The model under review builds one solid part; all positions refer to its coordinate system, in mm. A direction names the side the tool comes from. Give positions to 0.01 mm unless a question says otherwise; leave off trailing zeros. Loops run counter-clockwise (first coordinate to the right, second up) from the corner with the lowest first, then second, coordinate; pieces in that order, holes last. Notation, with made-up numbers: M 59.5,45.25 L 108.5,45.25 A26 ccw 108.5,65.25 Z; hole C 12,74.25 d10. An arc over 180 degrees is marked long. One line per item, written item: value. Start each with the question number.
Q1. We need section B-B on x = 0. Write out the cut boundary in (y, z), plus the area to 3 significant figures.
Q2. We need section C-C on z = -78. Write out the cut boundary in (x, y), plus the area to 3 significant figures.
Q3. For faces 1 (the face through (-41.09, -8.87, -68.35)), 2 (the face through (-61, -48, -85)), 3 (the face through (4.1, -9, 20)), 4 (the face through (0, -12, -7)), list the 3-axis set-ups (+Z, -Z, +X, -X, +Y, -Y) from which the entire face can be reached by the end or side of a thin tool; tool diameter is ignored.
Q4. To check wall thickness, follow line 1 along Y through (x, z) = (-46.5, -81); line 2 along X through (y, z) = (-4.55, 19.5); line 3 along Y through (x, z) = (0, 3.5). State the ranges of each line that lie inside material, in increasing order. Write a range as from..to.
Q5. Mouldability with a two-part tool opening along Y and no side actions: class faces 5 (the face through (0, -5, 30)), 6 (the face through (-61, -30, -85)), 7 (the face through (-7, 0, -22)), 8 (the face through (-41.09, -68.87, -68.35)) as released by +Y, released by -Y, zero draft, split by the parting line, or undercut.
Q6. We need section A-A on z = 19.5. Write out the cut boundary in (x, y).
Q7. We need section D-D on y = -9. Write out the cut boundary in (x, z).
Q8. For pin 1 (2 mm diameter, centred on x = -39.5, y = -53.5, fed in from -Z); pin 2 (17.5 mm diameter, centred on x = -4, y = -33.5, fed in from +Z); pin 3 (22 mm diameter, centred on x = -58, z = -84, fed in from +Y); pin 4 (2 mm diameter, centred on x = 0, z = 15.5, fed in from -Y), all flat-tipped, find the tip position at first contact; note any pin that passes through.
```python
from build123d import *

# Parameters (mm, degrees)
SKETCH_1_W          = 16
SKETCH_1_H          = 60
EXTRUDE_1_DEPTH     = 12
EXTRUDE_2_DEPTH     = 90
SKETCH_3_W          = 16
SKETCH_3_H          = 18
CUT_EXTRUDE_2_DEPTH = 50
CUT_EXTRUDE_START   = -6
SKETCH_2_W          = 8.2
SKETCH_2_H          = 20
SKETCH_2_R          = 1.75
CUT_EXTRUDE_3_DEPTH = 6
SKETCH_2_4_R        = 1.75
CUT_EXTRUDE_4_DEPTH = 12


with BuildPart() as part:
    # Sketch 1 → Extrude 1 (new body)
    with BuildSketch(Plane(origin=(0, 0, 0), x_dir=(1, 0, 0), z_dir=(0, 1, 0))):
        Rectangle(SKETCH_1_W, SKETCH_1_H)
    extrude(amount=-EXTRUDE_1_DEPTH)

    # Sketch 1_4 → Extrude 2 (add)
    with BuildSketch(Plane(origin=(0, 0, 0), x_dir=(1, 0, 0), z_dir=(0, 1, 0))):
        Polygon((-84.604444312, 94.278760969), (-74.319842557, 106.535472059), (2.284601755, 42.25671109), (-8, 30), align=None)
        with BuildLine():
            Line((-8, 30), (8, 30))
            ThreePointArc((8, 30), (6.500924593, 36.761892188), (2.284601755, 42.25671109))
            Line((2.284601755, 42.25671109), (-8, 30))
        make_face()
    extrude(amount=-EXTRUDE_2_DEPTH)

    # Sketch 3 → Cut-Extrude 2 (cut)
    with BuildSketch(Plane(origin=(-96.071153318, 0, -80.613269316), x_dir=(-0.64278761, 0, 0.766044443), z_dir=(-0.766044443, 0, -0.64278761))):
        with Locations((-25.839032416, -9)):
            Rectangle(SKETCH_3_W, SKETCH_3_H)
        with Locations((-25.839032416, -39)):
            Rectangle(SKETCH_3_W, SKETCH_3_H)
        with Locations((-25.839032416, -69)):
            Rectangle(SKETCH_3_W, SKETCH_3_H)
    extrude(amount=-CUT_EXTRUDE_2_DEPTH, mode=Mode.SUBTRACT)

    # Sketch 2 → Cut-Extrude 3 (cut)
    with BuildSketch(Plane(origin=(0, 0, 0), x_dir=(1, 0, 0), z_dir=(0, 1, 0)).offset(CUT_EXTRUDE_START)):
        with Locations((0, -20)):
            Rectangle(SKETCH_2_W, SKETCH_2_H)
        with Locations((0, -19.5)):
            Circle(SKETCH_2_R, mode=Mode.SUBTRACT)
        with Locations((0, -15.5)):
            Circle(SKETCH_2_R, mode=Mode.SUBTRACT)
    extrude(amount=-CUT_EXTRUDE_3_DEPTH, mode=Mode.SUBTRACT)

    # Sketch 2_4 → Cut-Extrude 4 (cut)
    with BuildSketch(Plane(origin=(0, 0, 0), x_dir=(1, 0, 0), z_dir=(0, 1, 0))):
        with Locations((0, -19.5)):
            Circle(SKETCH_2_4_R)
        with Locations((0, -15.5)):
            Circle(SKETCH_2_4_R)
    extrude(amount=-CUT_EXTRUDE_4_DEPTH, mode=Mode.SUBTRACT)


solid = part.part
```
Solved:
1. outline: M -90,-44.17 L 0,-44.17 L 0,13.75 L -6,13.75 L -6,10 L -12,10 L -12,-30 L -90,-30 Z; M -6,17.25 L 0,17.25 L 0,17.75 L -6,17.75 Z; M -6,21.25 L 0,21.25 L 0,30 L -6,30 Z
1. area: 1,830 mm2
2. outline: M -65.2,-90 L -40.31,-90 L -40.31,-78 L -65.2,-78 Z; M -65.2,-60 L -40.31,-60 L -40.31,-48 L -65.2,-48 Z; M -65.2,-30 L -40.31,-30 L -40.31,-18 L -65.2,-18 Z
2. area: 896 mm2
3. face 1: -Z, -X, +Y
3. face 2: -Z, -X
3. face 3: +Z, -Y
3. face 4: +Z, +X, -X, -Y
4. line 1: -90..-78, -60..-48, -30..-18
4. line 2: -8..-1.75, 1.75..8
4. line 3: -12..0
5. face 5: zero draft
5. face 6: undercut
5. face 7: released by +Y
5. face 8: undercut
6. outline: M -8,-12 L -4.1,-12 L -4.1,-6 L -1.75,-6 L -1.75,0 L -8,0 Z; M 1.75,-6 L 4.1,-6 L 4.1,-12 L 8,-12 L 8,0 L 1.75,0 Z
7. outline: M -46.3,-62.14 L -36.02,-74.4 L 2.28,-42.26 A16 ccw 8,-30 L 8,30 L 4.1,30 L 4.1,10 L -4.1,10 L -4.1,30 L -8,30 L -8,-30 Z
8. pin 1: z = -78.16
8. pin 2: z = -30
8. pin 3: y = -18
8. pin 4: through
